from build123d import *

# Parameters (mm, degrees)
F0_W     = 116.84
F0_H     = 114.3
F1_DEPTH = 76.2
F2_R     = 12.7
F2_R_2   = 19.05
F3_DEPTH = 25.4


with BuildPart() as f1:
    # F0 (on Front) → F1 (new body)
    with BuildSketch(Plane.XZ):
        with Locations((7.62, -19.05)):
            Rectangle(F0_W, F0_H)
    extrude(amount=F1_DEPTH)

    # F2 (on face) → F3 (cut)
    with BuildSketch(Plane.XZ.offset(76.2)):
        with Locations((13.195288, 3.787711)):
            Circle(F2_R)
        with Locations((34.671844, -42.966176)):
            Circle(F2_R_2)
        with Locations((-24.978266, -39.769248)):
            Circle(F2_R_2)
    extrude(amount=-F3_DEPTH, mode=Mode.SUBTRACT)


solid = f1.part
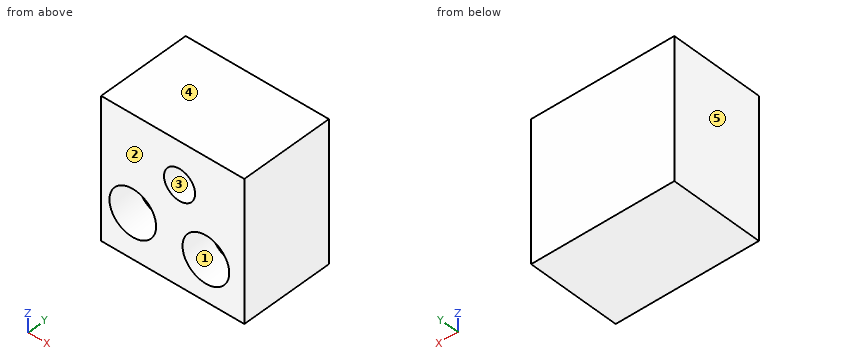
Verification items for the finished model (mm, model axes). Face numbers are marked on the shaded views. A direction names the side the tool comes from. Give positions to 0.01 mm unless a question says otherwise; leave off trailing zeros. Loops run counter-clockwise (first coordinate to the right, second up) from the corner with the lowest first, then second, coordinate; pieces in that order, holes last. Notation, with made-up numbers: (-21, 14.25) - (-13, 14.25) arc R21 cw to (-13, 19.25) - close; hole circle Ø7 at (48, 24). An arc over 180 degrees is marked (long way). Write each question's results on one line, items separated by ' | '.
1) Sectioned sample at A-A on y = -64.5. Record the boundary of the cut face in (x, z), plus the area to 3 significant figures.
Solution:
outline: (-50.8, -76.2) - (66.04, -76.2) - (66.04, 38.1) - (-50.8, 38.1) - close; hole circle Ø38.1 at (-24.98, -39.77); hole circle Ø25.4 at (13.2, 3.79); hole circle Ø38.1 at (34.67, -42.97) | area: 10,600 mm2
2) Sectioned sample at B-B on x = -42.5. Record the boundary of the cut face in (y, z).
Solution:
outline: (-76.2, -76.2) - (0, -76.2) - (0, 38.1) - (-76.2, 38.1) - (-76.2, -32.29) - (-50.8, -32.29) - (-50.8, -47.25) - (-76.2, -47.25) - close
3) Tool access check on the marked faces 1 and 2. Record the directions out of +Z, -Z, +X, -X, +Y, -Y that give a thin tool (end or side, any length) a straight path to the whole face; none if there is none.
Solution:
face 1: -Y | face 2: +Z, -Z, +X, -X, -Y
4) Depth check by flat-ended pin: P1, Ø3, axis at x = -19.5, z = -48.5, coming from the -Y side. Enter the tip coordinate at first touch or a pass-through.
Solution:
P1: y = -50.8
5) Sectioned sample at D-D on z = -56.5. Record the boundary of the cut face in (x, y), plus the area to 3 significant figures.
Solution:
outline: (-50.8, -76.2) - (-34.09, -76.2) - (-34.09, -50.8) - (-15.87, -50.8) - (-15.87, -76.2) - (21.27, -76.2) - (21.27, -50.8) - (48.08, -50.8) - (48.08, -76.2) - (66.04, -76.2) - (66.04, 0) - (-50.8, 0) - close | area: 7,760 mm2
6) Sectioned sample at C-C on z = -4.5. Record the boundary of the cut face in (x, y), plus the area to 3 significant figures.
Solution:
outline: (-50.8, -76.2) - (3.57, -76.2) - (3.57, -50.8) - (22.82, -50.8) - (22.82, -76.2) - (66.04, -76.2) - (66.04, 0) - (-50.8, 0) - close | area: 8,410 mm2
7) Material ranges on L1, parallel to X at y = -67, z = -29; L2, parallel to X at y = -51, z = -45; L3, parallel to Z at x = 3.5, y = -55, recorded low to high. Write a range as from..to.
Solution:
L1: -50.8..-40.69, -9.26..21.72, 47.63..66.04 | L2: -50.8..-43.3, -6.66..15.73, 53.61..66.04 | L3: -76.2..-4.42, 11.99..38.1
8) Mould release check, pull along Z, two halves, no side actions. Record for the marked faces 3, 4 and 5: pulls with the +Z half, pulls with the -Z half, needs draft (parallel to the pull), parting line crosses it, or undercut.
Solution:
face 3: undercut | face 4: pulls with the +Z half | face 5: needs draft
